The listing builds one solid part. Answer for the finished solid, in the listing's coordinates (mm). Face numbers are marked on the shaded views. A direction names the side the tool comes from. Coordinates: 2 decimals unless noted, no trailing zeros. Order: outer loops, then holes, each group sorted by start corner. A loop starts at its lowest first (then second) coordinate and runs counter-clockwise, first axis right, second up. Notation, with made-up numbers: (11, 49) -> (62, 49) arc R14 cw to (62, 72) -> close; hole circle Ø4 at (1, -20). An arc over 180 degrees is marked (long way). Return JSON: item names as keys, results as strings.
Autodesk Inventor part; units mm, degrees
ref_plane "YZ Plane" through (0, 0, 0) normal (1, 0, 0) x (0, 1, 0)
ref_plane "XZ Plane" through (0, 0, 0) normal (0, 1, 0) x (-1, 0, 0)
ref_plane "XY Plane" through (0, 0, 0) normal (0, 0, 1) x (1, 0, 0)
sketch "Sketch1" plane through (0, 0, 0) normal (0, 1, 0) x (-1, 0, 0)
  line L0 (0, 0) -> (-42, 0)
  line L1 (-42, 0) -> (-42, -24)
  line L2 (-42, -24) -> (24, -24)
  line L3 (24, -24) -> (24, 60)
  line L4 (24, 60) -> (0, 60)
  line L5 (0, 60) -> (0, 0)
  dimension "d0" = 24
  dimension "d1" = 42
  dimension "d2" = 24
  dimension "d3" = 60
extrude "Extrusion1" add sketch "Sketch1" along normal blind 42
sketch "Sketch2" plane through (0, 0, 0) normal (0, 0, 1) x (1, 0, 0)
  circle A0 centre (5.5, 36.5) radius 1.75
  circle A1 centre (36.5, 36.5) radius 1.75
  circle A2 centre (36.5, 5.5) radius 1.75
  circle A3 centre (5.5, 5.5) radius 1.75
  line L0 (42, 0) -> (42, 42)
  line L1 (0, 42) -> (42, 42)
  point P0 (0, 0)
  dimension "d6" = 3.5
  dimension "d7" = 5.5
  dimension "d8" = 5.5
  dimension "d9" = 31
  dimension "d10" = 31
extrude "Extrusion2" cut sketch "Sketch2" against normal blind 42
sketch "Sketch3" plane through (0, 0, 60) normal (1, 0, 0) x (0, 0, -1)
  circle A0 centre (12, 30) radius 5
  circle A1 centre (30, 12) radius 5
  circle A2 centre (48, 30) radius 5
  line L0 (12, 30) -> (30, 12) construction
  line L1 (30, 12) -> (48, 30) construction
  line L2 (0, 42) -> (60, 42) construction
  line L3 (0, 0) -> (0, 42) construction
  line L4 (0, 0) -> (60, 0) construction
  line L5 (60, 0) -> (60, 42) construction
  dimension "d13" = 12
  dimension "d14" = 12
  dimension "d15" = 12
  dimension "d16" = 10
  dimension "d17" = 12
sketch "Sketch4" plane through (-24, 0, -24) normal (-1, 0, 0) x (0, 0, 1)
  circle A0 centre (54, 12) radius 5
  circle A1 centre (36, 30) radius 5
  circle A2 centre (72, 30) radius 5
  circle A3 centre (54, 12) radius 3
  circle A4 centre (36, 30) radius 3
  circle A5 centre (72, 30) radius 3
  point P0 (24, 0)
  dimension "d20" = 6
extrude "Extrusion3" cut sketch "Sketch4" against normal blind 11 contours A0 | A1 | A2 | A3 | A4 | A5
extrude "Extrusion4" cut sketch "Sketch4" against normal blind 32.5 contours A3 | A4 | A5
sketch "Sketch6" plane through (0, 0, 0) normal (0, 0, 1) x (1, 0, 0)
  circle A0 centre (36.5, 5.5) radius 1.75 construction
  circle A1 centre (5.5, 5.5) radius 1.75 construction
  circle A2 centre (5.5, 36.5) radius 1.75 construction
  circle A3 centre (36.5, 36.5) radius 1.75 construction
  circle A4 centre (36.5, 5.5) radius 3
  circle A5 centre (5.5, 5.5) radius 3
  circle A6 centre (5.5, 36.5) radius 3
  circle A7 centre (36.5, 36.5) radius 3
  point P0 (0, 0)
  dimension "d23" = 6
extrude "Extrusion5" cut sketch "Sketch6" against normal blind 10
chamfer "Chamfer1" distance 1.25 angle 45 4 edges at (3.75, 5.5, -10) (3.75, 36.5, -10) (34.75, 36.5, -10) (34.75, 5.5, -10)
chamfer "Chamfer2" distance 0.5 angle 45 7 edges at (33.5, 5.5, 0) (2.5, 5.5, 0) (2.5, 36.5, 0) (33.5, 36.5, 0) (-24, 12, 25) (-24, 30, 7) (-24, 30, 43)
chamfer "Chamfer3" distance 3.5 angle 45 1 edges at (-24, 21, -24)
properties part number "XaxisMotorMount_3DPrint"
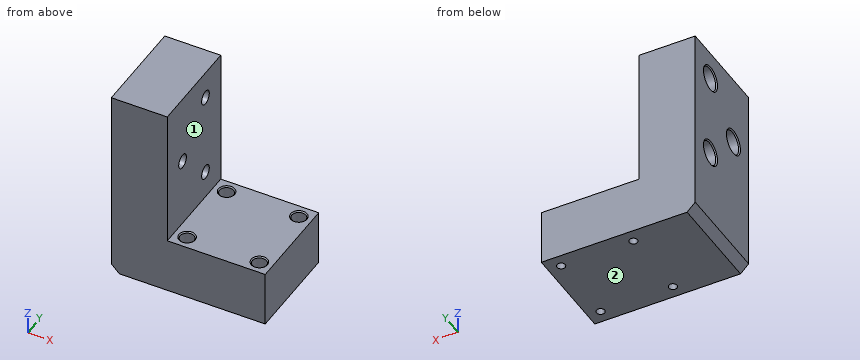
1. Each of these flat-tipped pins is pushed along its axis until it touches: pin 1 Ø5 at (y, z) = (29, 46) entering from +X; pin 2 Ø4 at (x, y) = (29, 10) entering from +Z; pin 3 Ø5.5 at (x, y) = (36.5, 5.5) entering from +Z. Where does it stop, or does it pass through?
Answer block:
{"pin 1": "stops at x = 0", "pin 2": "stops at z = 0", "pin 3": "stops at z = -10.25"}
2. The part is cut by section A-A on x = 5.5. Give the number of separate pieces and of enclosed holes in the cut face, and give its area (3 significant figures).
Answer block:
{"separate pieces": "3", "enclosed holes": "0", "area": "786 mm2"}
3. The part is cut by section D-D on z = 12. Give the vertices of the cut face in (x, y).
Answer block:
{"outline": "(-24, 0) -> (0, 0) -> (0, 27) -> (-13, 27) -> (-13, 25) -> (-23.5, 25) -> (-24, 24.5) -> close; (-24, 35.5) -> (-23.5, 35) -> (-13, 35) -> (-13, 33) -> (0, 33) -> (0, 42) -> (-24, 42) -> close"}
4. The part is cut by section B-B on y = 30. Give the vertices of the cut face in (x, z).
Answer block:
{"outline": "(-24, -20.5) -> (-20.5, -24) -> (42, -24) -> (42, 0) -> (0, 0) -> (0, 9) -> (-13, 9) -> (-13, 7) -> (-23.5, 7) -> (-24, 6.5) -> close; (-24, 17.5) -> (-23.5, 17) -> (-13, 17) -> (-13, 15) -> (0, 15) -> (0, 45) -> (-13, 45) -> (-13, 43) -> (-23.5, 43) -> (-24, 42.5) -> close; (-24, 53.5) -> (-23.5, 53) -> (-13, 53) -> (-13, 51) -> (0, 51) -> (0, 60) -> (-24, 60) -> close"}
5. For the marked faces 1 and 2, determine the directions among +Z, -Z, +X, -X, +Y, -Y from which every point of the face is accessible in a straight line to the end or side of a thin tool.
Answer block:
{"face 1": "+Z, +X, +Y, -Y", "face 2": "-Z, +X, -X, +Y, -Y"}
6. The part is cut by section C-C on y = 12. Give the vertices of the cut face in (x, z), and give its area (3 significant figures).
Answer block:
{"outline": "(-24, -20.5) -> (-20.5, -24) -> (42, -24) -> (42, 0) -> (0, 0) -> (0, 27) -> (-13, 27) -> (-13, 25) -> (-23.5, 25) -> (-24, 24.5) -> close; (-24, 35.5) -> (-23.5, 35) -> (-13, 35) -> (-13, 33) -> (0, 33) -> (0, 60) -> (-24, 60) -> close", "area": "2,830 mm2"}
7. Consider line 1 (Y direction, x = 36.5, z = -17.5); line 2 (Y direction, x = 5.5, z = -6.25); line 3 (X direction, y = 36, z = -7). Determine where each line is inside the solid, lowest interval first. Write a range as from..to.
Answer block:
{"line 1": "y = 0..3.75, 7.25..34.75, 38.25..42", "line 2": "y = 0..2.5, 8.5..33.5, 39.5..42", "line 3": "x = -24..2.54, 8.46..33.54, 39.46..42"}
